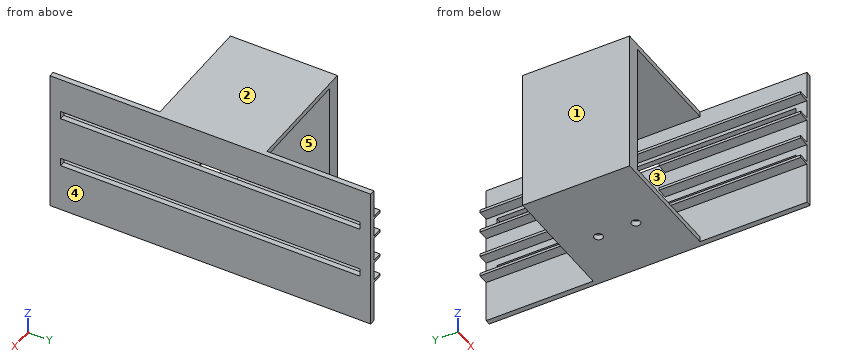
Autodesk Inventor part; units mm, degrees
ref_plane "YZ Plane" through (0, 0, 0) normal (1, 0, 0) x (0, 1, 0)
ref_plane "XZ Plane" through (0, 0, 0) normal (0, 1, 0) x (-1, 0, 0)
ref_plane "XY Plane" through (0, 0, 0) normal (0, 0, 1) x (1, 0, 0)
sketch "スケッチ1" plane through (0, 0, 0) normal (1, 0, 0) x (0, 1, 0)
  line L0 (60, -13.675) -> (-60, -13.675)
  line L1 (-60, -13.675) -> (-60, 13.675)
  line L2 (-60, 13.675) -> (60, 13.675)
  line L3 (60, 13.675) -> (60, -13.675)
  line L4 (60, -13.675) -> (-60, 13.675) construction
  line L5 (-60, -13.675) -> (60, 13.675) construction
  line L6 (-56, 11.258) -> (56, 11.258)
  line L7 (56, 11.258) -> (56, 8.258)
  line L8 (56, 8.258) -> (-56, 8.258)
  line L9 (-56, 8.258) -> (-56, 11.258)
  line L10 (-56, -8.258) -> (56, -8.258)
  line L11 (56, -8.258) -> (56, -11.258)
  line L12 (56, -11.258) -> (-56, -11.258)
  line L13 (-56, -11.258) -> (-56, -8.258)
  line L14 (60, -13.675) -> (-60, -13.675)
  line L15 (-60, -13.675) -> (-60, -29.5)
  line L16 (-60, -29.5) -> (60, -29.5)
  line L17 (60, -29.5) -> (60, -13.675)
  line L18 (-60, 13.675) -> (60, 13.675)
  line L19 (60, 13.675) -> (60, 24.5)
  line L20 (60, 24.5) -> (-60, 24.5)
  line L21 (-60, 24.5) -> (-60, 13.675)
  point P0 (0, 0)
  point P1 (0, 0)
  point P2 (56, 9.758)
  point P3 (56, -9.758)
  point P4 (0, 0)
  dimension "d1" = 120
  dimension "d3" = 9.758
  dimension "d6" = 3
  dimension "d11" = 9.758
  dimension "d15" = 2.417
  dimension "d26" = 4
  dimension "d27" = 4
  dimension "d41" = 29.5
  dimension "d53" = 54
extrude "押し出し1" add sketch "スケッチ1" along normal blind 2
sketch "スケッチ3" plane through (0, 0, 0) normal (-1, 0, 0) x (0, 0, 1)
  line L0 (-29.5, 60) -> (24.5, 60)
  line L1 (5.575, 60) -> (4.575, 60)
  line L2 (4.575, 60) -> (4.575, 7)
  line L3 (4.575, 7) -> (5.575, 7)
  line L4 (5.575, 7) -> (5.575, 60)
  line L5 (13.675, 60) -> (12.675, 60)
  line L6 (12.675, 60) -> (12.675, 0)
  line L7 (12.675, 0) -> (13.675, 0)
  line L8 (13.675, 0) -> (13.675, 60)
  line L9 (0, 0) -> (4.575, 0)
  line L10 (0, 0) -> (0, 19.0491)
  line L11 (5.575, -60) -> (4.575, -60)
  line L12 (4.575, -60) -> (4.575, -7)
  line L13 (4.575, -7) -> (5.575, -7)
  line L14 (5.575, -7) -> (5.575, -60)
  line L15 (13.675, -60) -> (12.675, -60)
  line L16 (12.675, -60) -> (12.675, 0)
  line L17 (13.675, 0) -> (13.675, -60)
  line L18 (-5.575, 60) -> (-4.575, 60)
  line L19 (-4.575, 60) -> (-4.575, 7)
  line L20 (-4.575, 7) -> (-5.575, 7)
  line L21 (-5.575, 7) -> (-5.575, 60)
  line L22 (-13.675, 60) -> (-12.675, 60)
  line L23 (-12.675, 60) -> (-12.675, 0)
  line L24 (-12.675, 0) -> (-13.675, 0)
  line L25 (-13.675, 0) -> (-13.675, 60)
  line L26 (-5.575, -60) -> (-4.575, -60)
  line L27 (-4.575, -60) -> (-4.575, -7)
  line L28 (-4.575, -7) -> (-5.575, -7)
  line L29 (-5.575, -7) -> (-5.575, -60)
  line L30 (-13.675, -60) -> (-12.675, -60)
  line L31 (-12.675, -60) -> (-12.675, 0)
  line L32 (-13.675, 0) -> (-13.675, -60)
  dimension "d31" = 1
  dimension "d33" = 1
  dimension "d34" = 60
  dimension "d35" = 7.1
  dimension "d36" = 7
  dimension "d54" = 13.675
extrude "押し出し4" add sketch "スケッチ3" along normal blind 4
sketch "スケッチ5" plane through (0, 0, 0) normal (-1, 0, 0) x (0, 0, 1)
  line L0 (-29.5, -60) -> (-29.5, 60)
  line L1 (-29.5, 20) -> (-27.5, 20)
  line L2 (-27.5, 20) -> (-27.5, -20)
  line L3 (-27.5, -20) -> (-29.5, -20)
  line L4 (-29.5, -20) -> (-29.5, 60)
  line L5 (24.5, 60) -> (24.5, -60)
  line L6 (24.5, 20) -> (22.5, 20)
  line L7 (22.5, 20) -> (22.5, -20)
  line L8 (22.5, -20) -> (24.5, -20)
  line L9 (24.5, -20) -> (24.5, 20)
  point P0 (0, 0)
  point P1 (-29.5, -20)
  dimension "d42" = 2
  dimension "d55" = 20
  dimension "d56" = 20
  dimension "d57" = 2
extrude "押し出し5" add sketch "スケッチ5" along normal blind 40
sketch "スケッチ6" plane through (2, -60, -29.5) normal (0, 0, -1) x (-1, 0, 0)
  circle A0 centre (20.75, 67) radius 1.6
  circle A1 centre (20.75, 53) radius 1.6
  line L0 (0, 0) -> (0, 120)
  point P0 (2, 60)
  point P1 (0, 60)
  dimension "d45" = 3.2
  dimension "d46" = 3.2
  dimension "d47" = 14
  dimension "d48" = 7
  dimension "d49" = 20.75
  dimension "d50" = 20.75
extrude "押し出し6" cut sketch "スケッチ6" against normal blind 2
sketch "スケッチ7" plane through (-40, 0, 0) normal (-1, 0, 0) x (0, 0, 1)
  line L0 (24.5, 20) -> (22.5, 20)
  line L1 (-29.5, 20) -> (-29.5, -20)
  line L2 (24.5, 20) -> (-29.5, 20)
  line L3 (-29.5, 20) -> (-29.5, -20)
  line L4 (-29.5, -20) -> (24.5, -20)
  line L5 (24.5, -20) -> (24.5, 20)
  point P0 (0, 0)
extrude "押し出し7" add sketch "スケッチ7" along normal blind 5
equation "\"d2\" = 0.25 * d0"
Build history of the part. All positions in model axes, mm. Face numbers are marked on the shaded views. A direction names the side the tool comes from. Coordinates: 2 decimals unless noted, no trailing zeros. Order: outer loops, then holes, each group sorted by start corner. A loop starts at its lowest first (then second) coordinate and runs counter-clockwise, first axis right, second up.
Item 1: Drill centre lines: L1, parallel to Y at x = -18.75, z = -28.25; L2, parallel to X at y = 6, z = -3.5; L3, parallel to Z at x = -22.5, y = 19. Where is each one in solid material? Low to high.
Filled in:
L1: y = -20 to -8.6, -5.4 to 5.4, 8.6 to 20
L2: x = -45 to -40, 0 to 2
L3: z = -29.5 to -27.5, 22.5 to 24.5
Item 2: Saw through at B-B on z = 7. List the corners of the cut face in (x, y), then the cut area to 3 significant figures.
Filled in:
outline: (-45, -20) - (-40, -20) - (-40, 20) - (-45, 20) - close; (0, -60) - (2, -60) - (2, 60) - (0, 60) - close
area: 440 mm2
Item 3: Saw through at D-D on x = -33. List the corners of the cut face in (y, z), then the cut area to 3 significant figures.
Filled in:
outline: (-20, -29.5) - (20, -29.5) - (20, -27.5) - (-20, -27.5) - close; (-20, 22.5) - (20, 22.5) - (20, 24.5) - (-20, 24.5) - close
area: 160 mm2
Item 4: Tool access for the marked faces 4 and 5: list every direction of +Z, -Z, +X, -X, +Y, -Y with a clear straight run to the whole face (end or side of a thin tool).
Filled in:
face 4: +Z, -Z, +X, +Y, -Y
face 5: +Y, -Y
Item 5: Drop flat-ended pins along their axis: pin 1 Ø2 at (x, y) = (-2.5, -26.5) entering from +Z (3 decimals); pin 2 Ø12 at (x, z) = (-35, 13.5) entering from -Y; pin 3 Ø22.5 at (x, z) = (-24, -9) entering from +Y. Give the stop position or say it passes through.
Filled in:
pin 1: stops at z = 13.675
pin 2: stops at y = -20
pin 3: passes through
Item 6: Saw through at A-A on x = -2.5. State how many separate pieces and enclosed holes the cut face has, then the cut area to 3 significant figures.
Filled in:
separate pieces: 8
enclosed holes: 0
area: 612 mm2
Item 7: Mould opens along Z. For the marked faces 1, 2 and 3 say: released by +Z, released by -Z, zero draft, split by the parting line, or undercut.
Filled in:
face 1: zero draft
face 2: released by +Z
face 3: undercut
